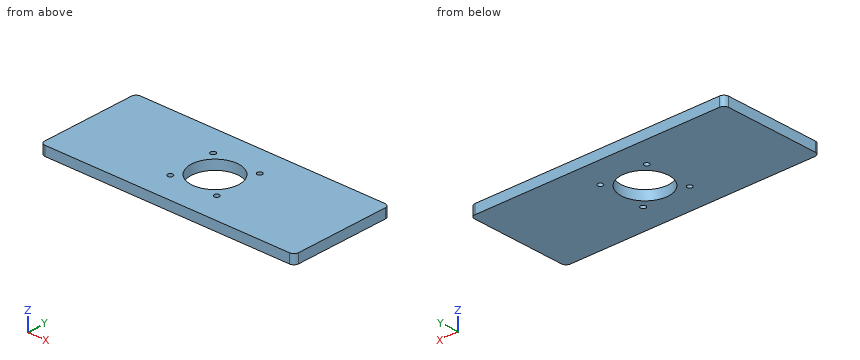
```python
from build123d import *

# Parameters (mm, degrees)
BOSS_EXTRUDE1_DEPTH  = 10
SKETCH2_R            = 25
CUT_EXTRUDE1_DEPTH   = 776.358804999
M5_CLEARANCE_HOLE1_D = 5.5


with BuildPart() as part:
    # Sketch1 → Boss-Extrude1 (new body)
    with BuildSketch(Plane.XY):
        with BuildLine():
            Line((-55, 50), (-55, -50))
            ThreePointArc((-55, -50), (-53.535533906, -53.535533906), (-50, -55))
            Line((-50, -55), (210, -55))
            ThreePointArc((210, -55), (213.535533906, -53.535533906), (215, -50))
            Line((215, -50), (215, 50))
            ThreePointArc((215, 50), (213.535533906, 53.535533906), (210, 55))
            Line((210, 55), (-50, 55))
            ThreePointArc((-50, 55), (-53.535533906, 53.535533906), (-55, 50))
        make_face()
    extrude(amount=BOSS_EXTRUDE1_DEPTH)

    # Sketch2 → Cut-Extrude1 (cut, through all)
    with BuildSketch(Plane(origin=(-479.845790405, 288.904934605, 10), x_dir=(1, 0, 0), z_dir=(0, 0, 1))):
        with Locations((559.845790405, -288.904934605)):
            Circle(SKETCH2_R)
    extrude(amount=-CUT_EXTRUDE1_DEPTH, mode=Mode.SUBTRACT)

    # M5 Clearance Hole1 (through all)
    with Locations(Plane(origin=(-479.845790405, 288.904934605, 10), x_dir=(1, 0, 0), z_dir=(0, 0, 1))):
        with Locations((535.097053063, -264.156197264), (584.594527746, -264.156197264), (584.594527746, -313.653671947), (535.097053063, -313.653671947)):
            Hole(M5_CLEARANCE_HOLE1_D / 2)


solid = part.part
```
Can you work these out from the model? Positions are in its coordinate system, mm. Give positions to 0.01 mm unless a question says otherwise; leave off trailing zeros. Write each loop counter-clockwise with the first axis right and the second up, starting at its lowest first coordinate (ties: lowest second). Pieces come first, ordered by that corner, then holes. Notation, with made-up numbers: (83, -30.5) - (99, -30.5) arc R27 ccw to (99, -2.5) - close; hole circle Ø3 at (-39.5, 13.5). An arc over 180 degrees is marked (long way). Write item = value, one per line. Start each with the question number.
1. Imagine slicing it at A-A (y = 0). Please give me the cut outline in (x, z), and give its area (3 significant figures).
2. For pin 1 (4.5 mm diameter, centred on x = 55.25, y = -24.75, fed in from -Z), with a flat end and sliding along its axis, tell me the tip position at first contact or that it passes through.
3. Imagine slicing it at B-B (x = 80). Please give me the cut outline in (y, z), and give its area (3 significant figures).
4. Please list where these lines run through material, in increasing order: line 1 (Y direction, x = 53, z = 2.25); line 2 (X direction, y = 26, z = 3.5); line 3 (Y direction, x = 80, z = 3).
5. Imagine slicing it at C-C (z = 3.5). Please give me the cut outline in (x, y).
Worked answers:
q1.outline = (-55, 0) - (55, 0) - (55, 10) - (-55, 10) - close; (105, 0) - (215, 0) - (215, 10) - (105, 10) - close
q1.area = 2,200 mm2
q2.pin_1 = through
q3.outline = (-55, 0) - (-25, 0) - (-25, 10) - (-55, 10) - close; (25, 0) - (55, 0) - (55, 10) - (25, 10) - close
q3.area = 600 mm2
q4.line_1 = -55 to -26.33, -23.17 to 23.17, 26.33 to 55
q4.line_2 = -55 to 52.8, 57.7 to 102.3, 107.2 to 215
q4.line_3 = -55 to -25, 25 to 55
q5.outline = (-55, -50) arc R5 ccw to (-50, -55) - (210, -55) arc R5 ccw to (215, -50) - (215, 50) arc R5 ccw to (210, 55) - (-50, 55) arc R5 ccw to (-55, 50) - close; hole circle Ø5.5 at (55.25, -24.75); hole circle Ø5.5 at (55.25, 24.75); hole circle Ø50 at (80, 0); hole circle Ø5.5 at (104.75, -24.75); hole circle Ø5.5 at (104.75, 24.75)
